from build123d import *

# Parameters (mm, degrees)
SKETCH_R     = 25
PAD_DEPTH    = 7
SKETCH001_W  = 5
SKETCH001_H  = 33.522271
PAD001_DEPTH = 25
FILLET_R     = 7
SKETCH002_R  = 1.5
POCKET_DEPTH = 35.301


with BuildPart() as part:
    # Sketch → Pad (new body)
    with BuildSketch(Plane.XY):
        Circle(SKETCH_R)
    extrude(amount=PAD_DEPTH)

    # Sketch001 → Pad001 (new body)
    with BuildSketch(Plane.XY.offset(7)):
        with Locations((7.8, -8.238865)):
            Rectangle(SKETCH001_W, SKETCH001_H)
    pad001 = extrude(amount=PAD001_DEPTH)

    # Mirrored: Pad001 across Sketch001 V_Axis
    add(pad001.mirror(Plane(origin=(0, 0, 7), x_dir=(0, 0, 1), z_dir=(1, 0, 0))))

    # Fillet
    fillet_edges = [part.edges().sort_by_distance(p)[0] for p in [
        (7.8, 8.522271, 32),
        (-7.8, 8.522271, 32),
    ]]
    fillet(fillet_edges, radius=FILLET_R)

    # Sketch002 → Pocket (cut, through all)
    with BuildSketch(Plane.YZ.offset(10.3)):
        with Locations((0, 13.956767)):
            Circle(SKETCH002_R)
        with Locations((-16.31287, 25.611097)):
            Circle(SKETCH002_R)
    extrude(amount=-POCKET_DEPTH, mode=Mode.SUBTRACT)


solid = part.part
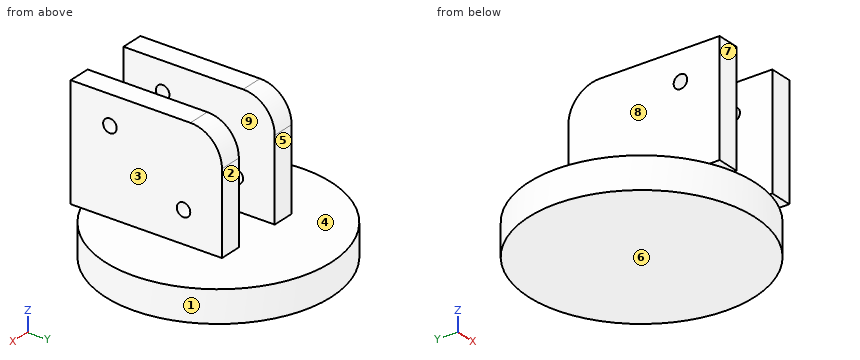
Source: CAD feature listing. Evaluate the final solid. Frame: model axes, mm. Face numbers are marked on the shaded views. A direction names the side the tool comes from. Give positions to 0.01 mm unless a question says otherwise; leave off trailing zeros. Loops run counter-clockwise (first coordinate to the right, second up) from the corner with the lowest first, then second, coordinate; pieces in that order, holes last. Notation, with made-up numbers: (22.5, 12) -> (44.5, 12) arc R30 cw to (44.5, 35) -> close; hole circle Ø4 at (-14, 80.5). An arc over 180 degrees is marked (long way). Use a Markdown table: item, result. Add a question column.
1) Line query: line 1 along Z through (x, y) = (7, 0); line 2 along X through (y, z) = (-21, 25.5); line 3 along Z through (x, y) = (3.5, -17.5). Output: solid intervals per line, ascending. Write a range as [from, to].
2) Section query D-D, the plane y = 6. Return the cut outline in (x, z).
3) Section query B-B, the plane y = 0. Return the cut outline in (x, z), then the cut area to 3 significant figures.
4) First-contact query: pin 1 (5 mm diameter, centred on x = -7, z = 22, fed in from +Y); pin 2 (12.5 mm diameter, centred on y = -14.5, z = 20, fed in from -X); pin 3 (1 mm diameter, centred on y = -16.5, z = 26.5, fed in from +X); pin 4 (3 mm diameter, centred on x = 14, y = 2.5, fed in from +Z). Flat tips, straight axial feed; report the tip coordinate or a pass-through.
5) Pull-direction query (X, two-part tool) for the marked faces 1, 2, 3 and 4; classes: +X half, -X half, draft (parallel to the pull), parting line (faces both ways), or undercut.
6) Section query A-A, the plane z = 22.5. Return the cut outline in (x, y).
7) Section query C-C, the plane x = 6. Return the cut outline in (y, z), then the cut area to 3 significant figures.
8) Reachability of the marked faces 5, 6, 7, 8 and 9 from +Z, -Z, +X, -X, +Y, -Y: full face, straight path, thin tool, end or side. Return the list, or none.
Numbers:
| question | item | result |
|---|---|---|
| 1 | line 1 | z = [0, 12.46], [15.46, 32] |
| 1 | line 2 | x = [-10.3, -5.3], [5.3, 10.3] |
| 1 | line 3 | z = [0, 7] |
| 2 | outline | (-24.27, 0) -> (24.27, 0) -> (24.27, 7) -> (10.3, 7) -> (10.3, 30.38) -> (5.3, 30.38) -> (5.3, 7) -> (-5.3, 7) -> (-5.3, 30.38) -> (-10.3, 30.38) -> (-10.3, 7) -> (-24.27, 7) -> close |
| 3 | outline | (-25, 0) -> (25, 0) -> (25, 7) -> (10.3, 7) -> (10.3, 12.46) -> (5.3, 12.46) -> (5.3, 7) -> (-5.3, 7) -> (-5.3, 12.46) -> (-10.3, 12.46) -> (-10.3, 7) -> (-25, 7) -> close; (-10.3, 15.46) -> (-5.3, 15.46) -> (-5.3, 32) -> (-10.3, 32) -> close; (5.3, 15.46) -> (10.3, 15.46) -> (10.3, 32) -> (5.3, 32) -> close |
| 3 | area | 570 mm2 |
| 4 | pin 1 | stops at y = 8.52 |
| 4 | pin 2 | stops at x = -10.3 |
| 4 | pin 3 | passes through |
| 4 | pin 4 | stops at z = 7 |
| 5 | face 1 | parting line |
| 5 | face 2 | draft |
| 5 | face 3 | +X half |
| 5 | face 4 | undercut |
| 6 | outline | (-10.3, -25) -> (-5.3, -25) -> (-5.3, 8.52) -> (-10.3, 8.52) -> close; (5.3, -25) -> (10.3, -25) -> (10.3, 8.52) -> (5.3, 8.52) -> close |
| 7 | outline | (-25, 7) -> (-24.27, 7) -> (-24.27, 0) -> (24.27, 0) -> (24.27, 7) -> (8.52, 7) -> (8.52, 25) arc R7 ccw to (1.52, 32) -> (-25, 32) -> close; hole circle Ø3 at (-16.31, 25.61); hole circle Ø3 at (0, 13.96) |
| 7 | area | 1,150 mm2 |
| 8 | face 5 | +Z, +X, -X, +Y |
| 8 | face 6 | -Z, +X, -X, +Y, -Y |
| 8 | face 7 | +Z, -Z, +X, -X, -Y |
| 8 | face 8 | +Z, -X, +Y, -Y |
| 8 | face 9 | +Z, +Y, -Y |
